Read the model definition and answer for the solid it produces. Units are mm, in the model's axes. Round coordinates to 2 decimals unless told otherwise and drop trailing zeros. Write each loop counter-clockwise with the first axis right and the second up, starting at its lowest first coordinate (ties: lowest second). Pieces come first, ordered by that corner, then holes.
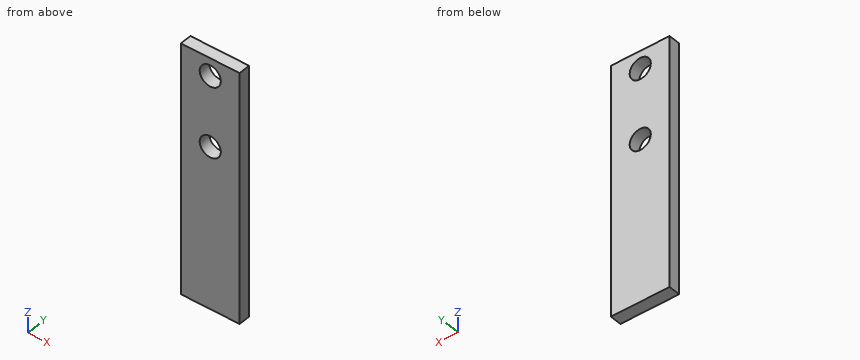
Autodesk Inventor part; units mm, degrees
ref_plane "YZ Plane" through (0, 0, 0) normal (1, 0, 0) x (0, 1, 0)
ref_plane "XZ Plane" through (0, 0, 0) normal (0, 1, 0) x (-1, 0, 0)
ref_plane "XY Plane" through (0, 0, 0) normal (0, 0, 1) x (1, 0, 0)
sketch "Sketch1" plane through (0, 0, 0) normal (0, 1, 0) x (-1, 0, 0)
  line L0 (-5, 21.25) -> (5, 21.25)
  line L1 (5, 21.25) -> (5, -21.25)
  line L2 (5, -21.25) -> (-5, -21.25)
  line L3 (-5, -21.25) -> (-5, 21.25)
  line L4 (-5, 21.25) -> (5, -21.25) construction
  line L5 (5, 21.25) -> (-5, -21.25) construction
  circle A0 centre (0, 6.25) radius 1.8
  circle A1 centre (0, 18.25) radius 1.8
  point P0 (0, 0)
  dimension "d0" = 42.5
  dimension "d1" = 10
  dimension "d4" = 15
  dimension "d5" = 3.6
  dimension "d27" = 3.6
  dimension "d28" = 3
extrude "Extrusion1" add sketch "Sketch1" along normal blind 2
sketch "Sketch2" plane through (0, 2, 0) normal (0, 1, 0) x (1, 0, 0)
  line L0 (-5.1166, 21.6617) -> (4.9098, 21.6617) construction
  line L1 (4.9098, 21.6617) -> (4.9098, -21.1785) construction
  line L2 (4.9098, -21.1785) -> (-5.1166, -21.1785) construction
  line L3 (-5.1166, -21.1785) -> (-5.1166, 21.6617) construction
  point P0 (0, 0)
decal "Decal1"
properties part number "sensorInferior"
Q1. Section C-C (y = 1.65) is taken. Determine the outline of the cut face in (x, z).
Verdict:
outline: (-5, -21.25) - (5, -21.25) - (5, 21.25) - (-5, 21.25) - close; hole circle Ø3.6 at (0, 6.25); hole circle Ø3.6 at (0, 18.25)
Q2. Section A-A (x = 0) is taken. Determine the outline of the cut face in (y, z).
Verdict:
outline: (0, -21.25) - (2, -21.25) - (2, 4.45) - (0, 4.45) - close; (0, 8.05) - (2, 8.05) - (2, 16.45) - (0, 16.45) - close; (0, 20.05) - (2, 20.05) - (2, 21.25) - (0, 21.25) - close
Q3. Straight lines are drawn through the part: probe 1 along Z at (x, y) = (0, 1.45); probe 2 along Z at (x, y) = (-1.25, 1.2); probe 3 along X at (y, z) = (1.35, 5). For each, find the intervals that lie inside material, in ascending order.
Verdict:
probe 1: z = -21.25 to 4.45, 8.05 to 16.45, 20.05 to 21.25
probe 2: z = -21.25 to 4.95, 7.55 to 16.95, 19.55 to 21.25
probe 3: x = -5 to -1.3, 1.3 to 5
Q4. Section B-B (z = 6.25) is taken. Determine the outline of the cut face in (x, y), then the cut area to 3 significant figures.
Verdict:
outline: (-5, 0) - (-1.8, 0) - (-1.8, 2) - (-5, 2) - close; (1.8, 0) - (5, 0) - (5, 2) - (1.8, 2) - close
area: 12.8 mm2
Q5. A flat-ended cylindrical pin translates along its axis: pin 1 Ø3 at (x, z) = (0, 6.25) entering from -Y. Find the tip coordinate at first contact, or state that the pin passes through.
Verdict:
pin 1: passes through
